Part model, mm, in its own coordinate system. A direction names the side the tool comes from. Give positions to 0.01 mm unless a question says otherwise; leave off trailing zeros. Loops run counter-clockwise (first coordinate to the right, second up) from the corner with the lowest first, then second, coordinate; pieces in that order, holes last. Notation, with made-up numbers: (62.5, 87) -> (107.5, 87) arc R36 cw to (107.5, 125) -> close; hole circle Ø10 at (68, 69.5). An arc over 180 degrees is marked (long way). Write item = value, one per line.
from build123d import *

# Parameters (mm, degrees)
SKETCH2_R           = 1.125
SKETCH2_W           = 2.12
SKETCH2_H           = 12.1
BOSS_EXTRUDE2_DEPTH = 2
BOSS_EXTRUDE3_DEPTH = 3
CHAMFER1_SIZE2      = 2
CHAMFER1_SIZE       = 5


with BuildPart() as part:
    # Sketch2 → Boss-Extrude2 (new body)
    with BuildSketch(Plane(origin=(0, 0, 0), x_dir=(1, 0, 0), z_dir=(0, 1, 0))):
        with BuildLine():
            Line((-10, 24.439438281), (-10, 17.439438281))
            Line((-10, 17.439438281), (10, 17.439438281))
            Line((10, 17.439438281), (10, 24.439438281))
            ThreePointArc((10, 24.439438281), (26.021613026, 19.342266443), (40, 10))
            Line((40, 10), (40, -10))
            Line((40, -10), (-40, -10))
            Line((-40, -10), (-40, 10))
            ThreePointArc((-40, 10), (-26.021613026, 19.342266443), (-10, 24.439438281))
        make_face()
        with Locations(Location((-37.490381057, -7.5, 0), (0, 0, 270))):
            Circle(SKETCH2_R, mode=Mode.SUBTRACT)
        with Locations(Location((37.490381057, -7.5, 0), (0, 0, 90))):
            Circle(SKETCH2_R, mode=Mode.SUBTRACT)
        with Locations(Location((-24.5, 15, 0), (0, 0, 270))):
            Circle(SKETCH2_R, mode=Mode.SUBTRACT)
        with Locations(Location((24.5, 15, 0), (0, 0, 90))):
            Circle(SKETCH2_R, mode=Mode.SUBTRACT)
        with Locations((15.56, 2.55)):
            Rectangle(SKETCH2_W, SKETCH2_H, mode=Mode.SUBTRACT)
        with Locations((-15.56, 2.55)):
            Rectangle(SKETCH2_W, SKETCH2_H, mode=Mode.SUBTRACT)
    extrude(amount=BOSS_EXTRUDE2_DEPTH)

    # Sketch3 → Boss-Extrude3 (add)
    with BuildSketch(Plane(origin=(0, 2, 0), x_dir=(1, 0, 0), z_dir=(0, 1, 0))):
        Polygon((12.419999998, -3.5), (37.42, -3.5), (37.42, 8.6), (12.419999998, 8.6), (12.419999998, 9.599999996), (38.419999998, 9.599999996), (38.419999998, -4.499999996), (12.419999998, -4.499999996), align=None)
        Polygon((-12.419999998, -3.5), (-12.419999998, -4.499999996), (-38.419999998, -4.499999996), (-38.419999998, 9.599999996), (-12.419999998, 9.599999996), (-12.419999998, 8.6), (-37.42, 8.6), (-37.42, -3.5), align=None)
    extrude(amount=BOSS_EXTRUDE3_DEPTH)

    # Chamfer1
    chamfer1_edges = [part.edges().sort_by_distance(p)[0] for p in [
        (0, 2, -17.439438281),
    ]]
    chamfer1_side = [part.faces().sort_by_distance(p)[0] for p in [
        (0, 2, -17.399438281),
    ]]
    chamfer(chamfer1_edges, length=CHAMFER1_SIZE - 0.0001, length2=CHAMFER1_SIZE2 - 0.0001, reference=chamfer1_side[0])  # a hair under: the kernel refuses the full size


solid = part.part
1) Pull direction Z, two halves, no side cores. Call faces 1 (the face through (1, 0, -4)), 2 (the face through (16.62, 1, -2)), 3 (the face through (26, 3, 4.5)): pulls with the +Z half, pulls with the -Z half, needs draft (parallel to the pull), parting line crosses it, or undercut.
Resolved:
face_1 = needs draft
face_2 = undercut
face_3 = pulls with the +Z half
2) Drop flat-ended pins along their axis: P1, Ø9.5, axis at x = -27, z = -3, coming from the +Y side; P2, Ø1.3, axis at x = 24.5, z = -15, coming from the -Y side; P3, Ø2.5, axis at x = -28.5, y = 4, coming from the +Z side; P4, Ø2, axis at y = 1, z = -19, coming from the -X side. Give the stop position or say it passes through.
Resolved:
P1 = 2
P2 = through
P3 = 4.5
P4 = -28.64
3) Slice it at B-B, the plane z = -21.5. List the corners of the cut face in (x, y).
Resolved:
outline = (-20.96, 0) -> (-10, 0) -> (-10, 2) -> (-20.96, 2) -> close; (10, 0) -> (20.96, 0) -> (20.96, 2) -> (10, 2) -> close
4) Which spindle directions (+Z, -Z, +X, -X, +Y, -Y) get a long thin tool onto all of the face, cutting with end or side? Do faces 4 (the face through (-26, 3, -9.6)), 5 (the face through (-25, 4, -8.6)), 6 (the face through (-10, 1, -20)). Say none if no direction does.
Resolved:
face_4 = -Z, +X, -X, +Y
face_5 = +Y
face_6 = -Z, +Y
5) Slice it at C-C, the plane y = 0.9. List the corners of the cut face in (x, z) (3 decimals).
Resolved:
outline = (-40, -10) arc R60 ccw to (-10, -24.439) -> (-10, -15.19) -> (10, -15.19) -> (10, -24.439) arc R60 ccw to (40, -10) -> (40, 10) -> (-40, 10) -> close; hole circle Ø2.25 at (-37.49, 7.5); hole circle Ø2.25 at (-24.5, -15); hole (-16.62, -8.6) -> (-14.5, -8.6) -> (-14.5, 3.5) -> (-16.62, 3.5) -> close; hole (14.5, -8.6) -> (16.62, -8.6) -> (16.62, 3.5) -> (14.5, 3.5) -> close; hole circle Ø2.25 at (24.5, -15); hole circle Ø2.25 at (37.49, 7.5)
6) Slice it at D-D, the plane x = 24.5. List the corners of the cut face in (y, z) (3 decimals), and give its area (3 significant figures).
Resolved:
outline = (0, -20.049) -> (2, -20.049) -> (2, -16.125) -> (0, -16.125) -> close; (0, -13.875) -> (2, -13.875) -> (2, -9.6) -> (5, -9.6) -> (5, -8.6) -> (2, -8.6) -> (2, 3.5) -> (5, 3.5) -> (5, 4.5) -> (2, 4.5) -> (2, 10) -> (0, 10) -> close
area = 61.6 mm²
7) Slice it at A-A, the plane z = 7.5. List the corners of the cut face in (x, y), and give its area (3 significant figures).
Resolved:
outline = (-40, 0) -> (-38.62, 0) -> (-38.62, 2) -> (-40, 2) -> close; (-36.37, 0) -> (36.37, 0) -> (36.37, 2) -> (-36.37, 2) -> close; (38.62, 0) -> (40, 0) -> (40, 2) -> (38.62, 2) -> close
area = 151 mm²
8) Drill centre lines: line 1 along X through (y, z) = (1.25, 7.5); line 2 along Z through (x, y) = (-19, 2.3); line 3 along X through (y, z) = (3.95, -6.5). Where is each one in solid material? Low to high. Write a range as [from, to].
Resolved:
line_1 = [-40, -38.62], [-36.37, 36.37], [38.62, 40]
line_2 = [-9.6, -8.6], [3.5, 4.5]
line_3 = [-38.42, -37.42], [37.42, 38.42]
